```python
from build123d import *

# Parameters (mm, degrees)
SKETCH_1_W          = 74
SKETCH_1_H          = 10
EXTRUDE_1_DEPTH     = 6
SKETCH_2_R          = 1.55
CUT_EXTRUDE_1_DEPTH = 10
SKETCH_3_R          = 2.5
SKETCH_3_R_2        = 1.55
EXTRUDE_2_DEPTH     = 3
FILLET_5_R          = 0.5
FILLET_7_R          = 0.5


with BuildPart() as part:
    # 草图1 → 凸台-拉伸1 (new body)
    with BuildSketch(Plane.XY):
        with Locations((12.900383142, 1.335145162)):
            Rectangle(SKETCH_1_W, SKETCH_1_H)
    extrude(amount=EXTRUDE_1_DEPTH)

    # 草图2 → 切除-拉伸1 (cut)
    with BuildSketch(Plane.XY.offset(6)):
        with Locations((-16.099616858, 1.335145162)):
            Circle(SKETCH_2_R)
        with Locations((41.900383142, 1.335145162)):
            Circle(SKETCH_2_R)
    extrude(amount=-CUT_EXTRUDE_1_DEPTH, mode=Mode.SUBTRACT)

    # 草图3 → 凸台-拉伸2 (add)
    with BuildSketch(Plane.XY.offset(6)):
        with Locations((-16.099616858, 1.335145162)):
            Circle(SKETCH_3_R)
        with Locations((-16.099616858, 1.335145162)):
            Circle(SKETCH_3_R_2, mode=Mode.SUBTRACT)
        with Locations((41.900383142, 1.335145162)):
            Circle(SKETCH_3_R)
        with Locations((41.900383142, 1.335145162)):
            Circle(SKETCH_3_R_2, mode=Mode.SUBTRACT)
    extrude(amount=EXTRUDE_2_DEPTH)

    # 圆角5
    fillet_5_edges = [part.edges().sort_by_distance(p)[0] for p in [
        (39.400383142, 1.335145162, 6),
    ]]
    fillet(fillet_5_edges, radius=FILLET_5_R)

    # 圆角7
    fillet_7_edges = [part.edges().sort_by_distance(p)[0] for p in [
        (-18.599616858, 1.335145162, 6),
    ]]
    fillet(fillet_7_edges, radius=FILLET_7_R)


solid = part.part
```
Model file for the job. Use its own axes, mm. A direction names the side the tool comes from. Coordinates: 2 decimals unless noted, no trailing zeros. Loops run counter-clockwise (first coordinate to the right, second up) from the corner with the lowest first, then second, coordinate; pieces in that order, holes last. Notation, with made-up numbers: (24, -6) - (69, -6) arc R31 cw to (69, 33) - close; hole circle Ø1 at (21.5, 21.5). An arc over 180 degrees is marked (long way). Answer as a JSON object with one key per item and string values. Group by question number.
(1) Flat gauge pin, fed straight in: pin 1 (3 mm diameter, centred on x = 18.5, y = 2, fed in from +Z). Where does the tip first touch, or does it go through?
(2) Cut at A-A (z = 4.5). Give the cut face in (x, y).
(3) Cut at C-C (y = -3). Give the cut face in (x, z), then the cut area to 3 significant figures.
(4) Tool access for faces 1 (the face through (-18.6, 1.4, 7.7)), 2 (the face through (-14, 1, 9)): list every direction of +Z, -Z, +X, -X, +Y, -Y with a clear straight run to the whole face (end or side of a thin tool).
(5) Two-plate mould, pull along X, no slides. Class faces 3 (the face through (12, -3.665, 3)), 4 (the face through (-24.1, 1, 3)), 5 (the face through (44.21, 0.38, 7.73)): released by +X, released by -X, zero draft, split by the parting line, or undercut.
(6) Cut at B-B (x = 32). Give the cut face in (y, z), then the cut area to 3 significant figures.
(7) Probe line 1 along Y through (x, z) = (42, 2.5); line 2 along X through (y, z) = (2.5, 2.25); line 3 along Z through (x, y) = (6.5, 0.25). List the from-to ranges inside material, lowest first.
Geometry says:
{
 "1": {"pin 1": "stops at z = 6"},
 "2": {"outline": "(-24.1, -3.66) - (49.9, -3.66) - (49.9, 6.34) - (-24.1, 6.34) - close; hole circle Ø3.1 at (-16.1, 1.34); hole circle Ø3.1 at (41.9, 1.34)"},
 "3": {"outline": "(-24.1, 0) - (49.9, 0) - (49.9, 6) - (-24.1, 6) - close", "area": "444 mm^2"},
 "4": {"face 1": "+Z", "face 2": "+Z, +X, -X, +Y, -Y"},
 "5": {"face 3": "zero draft", "face 4": "released by -X", "face 5": "undercut"},
 "6": {"outline": "(-3.66, 0) - (6.34, 0) - (6.34, 6) - (-3.66, 6) - close", "area": "60.0 mm^2"},
 "7": {"line 1": "y = -3.66 to -0.21, 2.88 to 6.34", "line 2": "x = -24.1 to -17.12, -15.08 to 40.88, 42.92 to 49.9", "line 3": "z = 0 to 6"}
}
